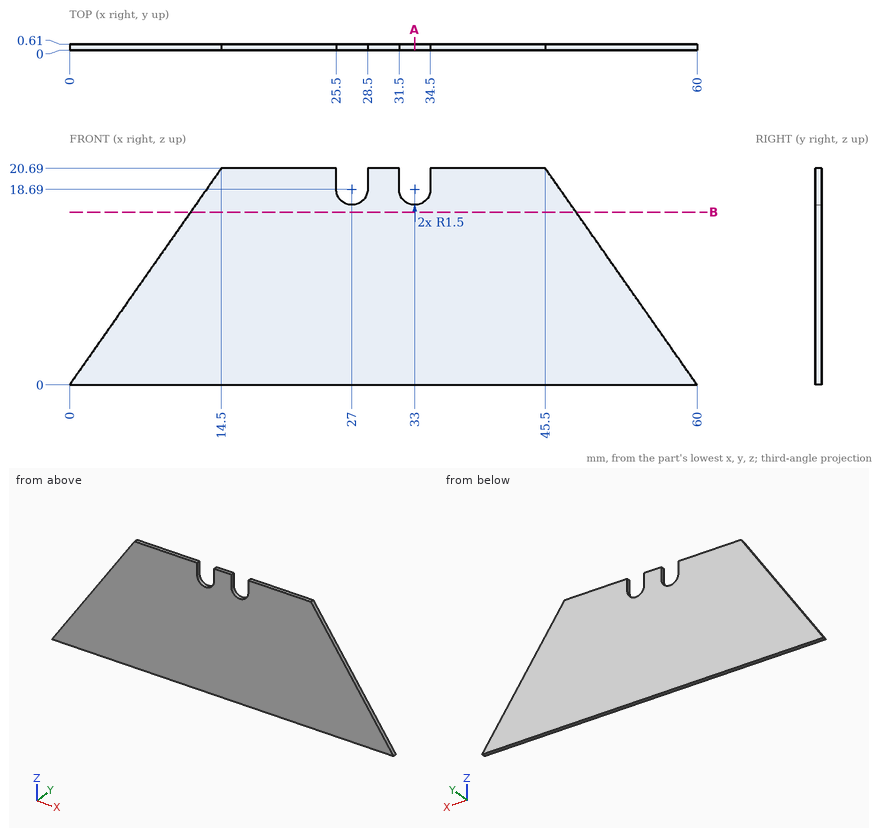
Job drawing, mm, ordinate dimensions from the low corner. One solid piece. Round coordinates to 2 decimals unless told otherwise and drop trailing zeros. Write each loop counter-clockwise with the first axis right and the second up, starting at its lowest first coordinate (ties: lowest second). Pieces come first, ordered by that corner, then holes. Notation, with made-up numbers: M -3,-11.5 L 21,-11.5 A17 ccw 21,3.5 Z; hole C -25.75,75.25 d8. An arc over 180 degrees is marked long. Return JSON: item names as keys, results as strings. Group by question number.
(1) Saw through at B-B on z = 16.5. Write the cut outline in (x, y).
(2) Drill centre lines: probe 1 along X at (y, z) = (0.05, 19) (1 decimal); probe 2 along X at (y, z) = (0.3, 8.75); probe 3 along Z at (x, y) = (7.5, 0.1). Where is each one in solid material? Low to high.
(3) Saw through at A-A on x = 33. Write the cut outline in (y, z), then the cut area to 3 significant figures.
Returned:
{
 "1": {"outline": "M 11.56,0 L 48.44,0 L 48.44,0.61 L 11.56,0.61 Z"},
 "2": {"probe 1": "13.3 to 25.5, 28.5 to 31.5, 34.5 to 46.7", "probe 2": "6.13 to 53.87", "probe 3": "0 to 10.7"},
 "3": {"outline": "M 0,0 L 0.61,0 L 0.61,17.19 L 0,17.19 Z", "area": "10.5 mm²"}
}
